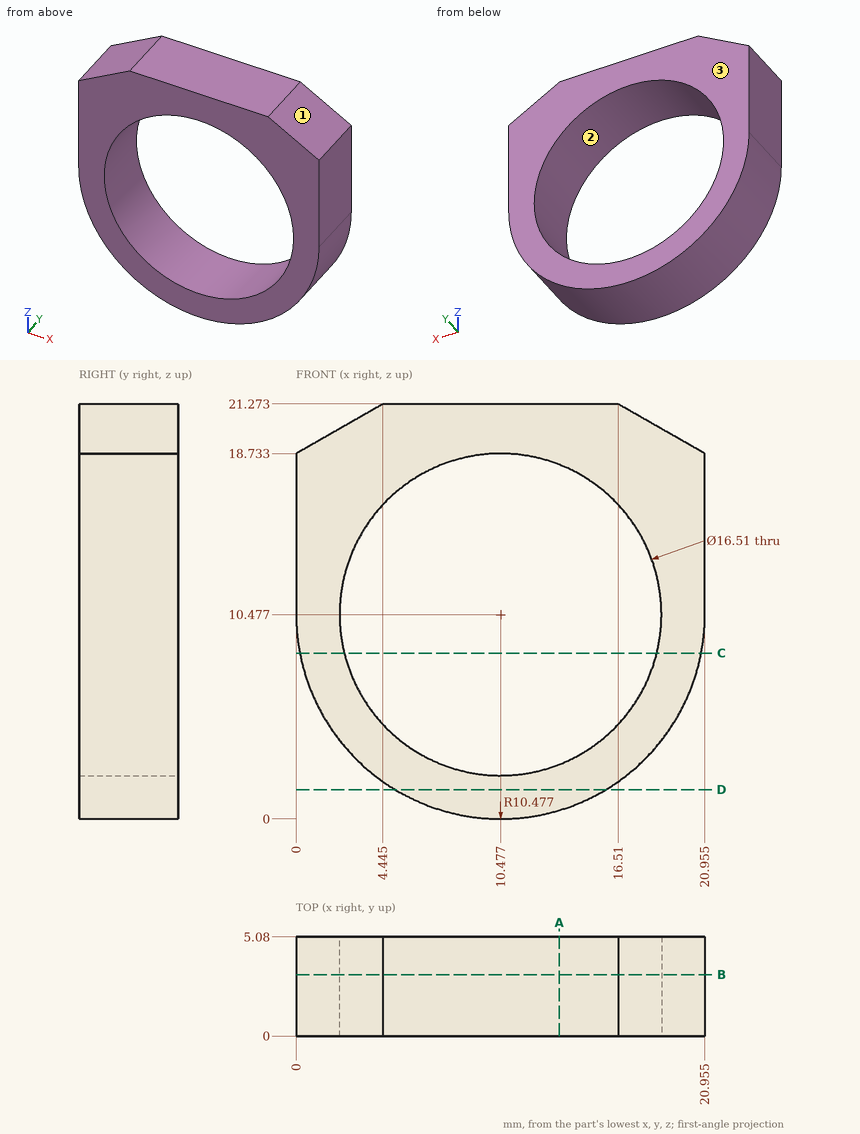
Verification items for this drawing (mm, ordinates from the low corner). Round coordinates to 2 decimals unless told otherwise and drop trailing zeros. Order: outer loops, then holes, each group sorted by start corner. A loop starts at its lowest first (then second) coordinate and runs counter-clockwise, first axis right, second up. Notation, with made-up numbers: (-3.5, 24.5) - (23.5, 24.5) arc R12 cw to (23.5, 47.5) - close; hole circle Ø2 at (63, 66). An arc over 180 degrees is marked (long way). Answer as CSV lines item,"result". Start each with the question number.
1) Draft check along X on the marked faces 1, 2 and 3. Enter one of: +X half, -X half, draft (parallel to the pull), parting line (faces both ways), or undercut.
2) Section check C-C (z = 8.5). Record the cut outline in (x, y), then the cut area to 3 significant figures.
3) Section check D-D (z = 1.5). Record the cut outline in (x, y) (1 decimal).
4) Section check B-B (y = 3.15). Record the cut outline in (x, z) (1 decimal).
5) Depth check by flat-ended pin: pin 1 (2 mm diameter, centred on x = 4.5, z = 11, fed in from +Y); pin 2 (2 mm diameter, centred on y = 2, z = 8.5, fed in from -X); pin 3 (1.5 mm diameter, centred on x = 5.5, y = 4, fed in from -Z). Enter the tip coordinate at first touch or a pass-through.
6) Scan lines: probe 1 along Z at (x, y) = (10.5, 4.7); probe 2 along X at (y, z) = (1.2, 16.25) (1 decimal); probe 3 along X at (y, z) = (1.85, 12) (1 decimal). Record each from-to range of solid material in increasing order.
7) Section check A-A (x = 13.5). Record the cut outline in (y, z) (1 decimal).
Determined:
1,face 1,"+X half"
1,face 2,"undercut"
1,face 3,"draft"
2,outline,"(0.19, 0) - (2.46, 0) - (2.46, 5.08) - (0.19, 5.08) - close; (18.49, 0) - (20.77, 0) - (20.77, 5.08) - (18.49, 5.08) - close"
2,area,"23.1 mm^2"
3,outline,"(5.1, 0) - (15.9, 0) - (15.9, 5.1) - (5.1, 5.1) - close"
4,outline,"(0, 10.5) arc R10.5 ccw to (21, 10.5) - (21, 18.7) - (16.5, 21.3) - (4.4, 21.3) - (0, 18.7) - close; hole circle Ø16.5 at (10.5, 10.5)"
5,pin 1,"through"
5,pin 2,"x = 0.05"
5,pin 3,"z = 0.89"
6,probe 1,"0 to 2.22, 18.73 to 21.27"
6,probe 2,"0 to 4.6, 16.4 to 21"
6,probe 3,"0 to 2.4, 18.6 to 21"
7,outline,"(0, 0.4) - (5.1, 0.4) - (5.1, 2.8) - (0, 2.8) - close; (0, 18.2) - (5.1, 18.2) - (5.1, 21.3) - (0, 21.3) - close"
